```python
from build123d import *
from build123d.topology import SkipClean

# Parameters (mm, degrees)
SKETCH2_R           = 2.5
BOSS_EXTRUDE1_DEPTH = 7
FILLET1_R           = 90
BOSS_EXTRUDE3_DEPTH = 15
SKETCH4_R           = 8
CUT_EXTRUDE1_DEPTH  = 10
BOSS_EXTRUDE4_START = 10
BOSS_EXTRUDE4_DEPTH = 10
BOSS_EXTRUDE5_DEPTH = 27
SKETCH7_R           = 2.5
CUT_EXTRUDE2_DEPTH  = 37
INTERSECT3_DEPTH    = 27


with BuildPart() as part:
    # Sketch2 → Boss-Extrude1 (new body)
    with BuildSketch(Plane(origin=(0, 0, 0), x_dir=(1, 0, 0), z_dir=(0, 1, 0))):
        with BuildLine():
            Line((-4.24846021, -9.602113613), (13.572308451, -17.486922065))
            ThreePointArc((13.572308451, -17.486922065), (20.638500285, -15.805826469), (20.907079545, -8.547382103))
            Line((20.907079545, -8.547382103), (11.451696022, 4.891208687))
            ThreePointArc((11.451696022, 4.891208687), (9.270724445, 7.034926316), (6.472222222, 8.268031175))
            ThreePointArc((6.472222222, 8.268031175), (4.86754966, 9.30359932), (3.101845071, 10.031378627))
            Line((3.101845071, 10.031378627), (-8.821699821, 13.718308443))
            ThreePointArc((-8.821699821, 13.718308443), (-15.091857172, 11.987583677), (-16.147811194, 5.569231667))
            Line((-16.147811194, 5.569231667), (-12.308520784, -3.358124948))
            ThreePointArc((-12.308520784, -3.358124948), (-9.971976629, -6.504419403), (-6.472222222, -8.268031175))
            ThreePointArc((-6.472222222, -8.268031175), (-5.401685102, -9.003987898), (-4.24846021, -9.602113613))
        make_face()
        with Locations(Location((16, -12, 0), (0, 0, 270))):
            Circle(SKETCH2_R, mode=Mode.SUBTRACT)
        with Locations(Location((-10.604337088, 7.953252816, 0), (0, 0, 270))):
            Circle(SKETCH2_R, mode=Mode.SUBTRACT)
        with BuildLine():
            ThreePointArc((-4.694444444, -4.495797077), (0, -6.5), (4.694444444, -4.495797077))
            ThreePointArc((4.694444444, -4.495797077), (9, 0), (4.694444444, 4.495797077))
            ThreePointArc((4.694444444, 4.495797077), (0, 6.5), (-4.694444444, 4.495797077))
            ThreePointArc((-4.694444444, 4.495797077), (-9, 0), (-4.694444444, -4.495797077))
        make_face(mode=Mode.SUBTRACT)
    extrude(amount=BOSS_EXTRUDE1_DEPTH)

    # Fillet1
    fillet1_edges = [part.edges().sort_by_distance(p)[0] for p in [
        (6.472222222, 3.5, -8.268031175),
        (-6.472222222, 3.5, 8.268031175),
    ]]
    fillet(fillet1_edges, radius=FILLET1_R)

    # Sketch3 → Boss-Extrude3 (add)
    with BuildSketch(Plane(origin=(0, 7, 0), x_dir=(1, 0, 0), z_dir=(0, 1, 0))):
        with BuildLine():
            Line((-13.446880098, 1.012795393), (-12.308520784, -3.358124948))
            ThreePointArc((-12.308520784, -3.358124948), (-10.611843956, -5.907229762), (-8.121968415, -7.689690813))
            ThreePointArc((-8.121968415, -7.689690813), (-6.480430757, -8.483296944), (-4.855306799, -9.309994408))
            ThreePointArc((-4.855306799, -9.309994408), (-4.554226262, -9.460920841), (-4.24846021, -9.602113613))
            Line((-4.24846021, -9.602113613), (-1.454246479, -10.838414946))
            ThreePointArc((-1.454246479, -10.838414946), (10.979115699, -7.880432641), (11.451696022, 4.891208687))
            ThreePointArc((11.451696022, 4.891208687), (9.968863726, 6.507036925), (8.121968415, 7.689690813))
            ThreePointArc((8.121968415, 7.689690813), (6.480430757, 8.483296944), (4.855306799, 9.309994408))
            ThreePointArc((4.855306799, 9.309994408), (3.994892398, 9.710346787), (3.101845071, 10.031378627))
            Line((3.101845071, 10.031378627), (-3.895223267, 11.305534387))
            ThreePointArc((-3.895223267, 11.305534387), (-5.691953988, 10.727471116), (-6.207623157, 8.911848981))
            ThreePointArc((-6.207623157, 8.911848981), (-7.30582589, 4.892236012), (-11.232333003, 3.497288147))
            ThreePointArc((-11.232333003, 3.497288147), (-13.004436636, 2.847636589), (-13.446880098, 1.012795393))
        make_face()
        with BuildLine():
            ThreePointArc((4.694444444, -4.495797077), (9, 0), (4.694444444, 4.495797077))
            ThreePointArc((4.694444444, 4.495797077), (0, 6.5), (-4.694444444, 4.495797077))
            ThreePointArc((-4.694444444, 4.495797077), (-9, 0), (-4.694444444, -4.495797077))
            ThreePointArc((-4.694444444, -4.495797077), (0, -6.5), (4.694444444, -4.495797077))
        make_face(mode=Mode.SUBTRACT)
    extrude(amount=BOSS_EXTRUDE3_DEPTH)

    # Sketch4 → Cut-Extrude1 (cut)
    with BuildSketch(Plane(origin=(0, 22, 0), x_dir=(1, 0, 0), z_dir=(0, 1, 0))):
        Circle(SKETCH4_R)
    extrude(amount=-CUT_EXTRUDE1_DEPTH, mode=Mode.SUBTRACT)

    # Sketch5 → Boss-Extrude4 (add)
    with SkipClean():  # the faces are left unmerged after this step: merging them gives an invalid solid
        with BuildSketch(Plane(origin=(0, 12, 0), x_dir=(1, 0, 0), z_dir=(0, 1, 0)).offset(BOSS_EXTRUDE4_START)):
            with BuildLine():
                ThreePointArc((-7.111111111, 3.664982778), (-8, 0), (-7.111111111, -3.664982778))
                ThreePointArc((-7.111111111, -3.664982778), (-9, 0), (-7.111111111, 3.664982778))
            make_face()
            with BuildLine():
                ThreePointArc((7.111111111, -3.664982778), (9, 0), (7.111111111, 3.664982778))
                ThreePointArc((7.111111111, 3.664982778), (8, 0), (7.111111111, -3.664982778))
            make_face()
        extrude(amount=-BOSS_EXTRUDE4_DEPTH)


with BuildPart() as body_2:
    # Sketch6 → Boss-Extrude5 (new body)
    with BuildSketch(Plane(origin=(0, 0, 0), x_dir=(-1, 0, 0), z_dir=(0, -1, 0))):
        Polygon((8.401052482, 26.937158796), (-31.729302738, -9.377746691), (-13.016359271, -30.388770935), (27.113995949, 5.926134553), align=None)
    extrude(amount=-BOSS_EXTRUDE5_DEPTH)

    # Sketch7 → Cut-Extrude2 (cut)
    with BuildSketch(Plane(origin=(-9.25873614, 0, 10.23151142), x_dir=(0.7414761288495602, 0, 0.670979247329059), z_dir=(-0.670979247329059, 0, 0.7414761288495602))):
        with Locations((-16.542969249, 20.228212297)):
            Circle(SKETCH7_R)
        with Locations((19.254983261, 20.228212297)):
            Circle(SKETCH7_R)
    extrude(amount=-CUT_EXTRUDE2_DEPTH, mode=Mode.SUBTRACT)

    # Intersect1: read off the stored shape, not the designer's step
    # Intersect1: cut part
    add(part.part, mode=Mode.SUBTRACT)

    # Intersect3: read off the stored shape, not the designer's step
    # Intersect3 outline → Intersect3 (cut)
    with BuildSketch(Plane(origin=(0, 0, 0), x_dir=(1, 0, 0), z_dir=(0, 1, 0))):
        Polygon((13.016359271, -30.388770935), (22.372831004, -19.883258813), (-17.757524216, 16.431646675), (-27.113995949, 5.926134553), align=None)
    extrude(amount=INTERSECT3_DEPTH, mode=Mode.SUBTRACT)


solid = body_2.part
```
Can you work these out from the model? Positions are in its coordinate system, mm. A direction names the side the tool comes from. Round coordinates to 2 decimals unless told otherwise and drop trailing zeros. Loops run counter-clockwise (first coordinate to the right, second up) from the corner with the lowest first, then second, coordinate; pieces in that order, holes last. Notation, with made-up numbers: (56, 32) -> (108, 32) arc R15 ccw to (108, 38) -> close; hole circle Ø6 at (19, -40). An arc over 180 degrees is marked (long way). One line per item, written item: value. Start each with the question number.
1. If we mould it in two halves opening along Y, with no side actions, what happens to faces 3 (the flat face through (7, 0, -9)), 4 (the cylindrical face through (17.735, 3.451, 10.2)), 5 (the cylindrical face through (-7.834, 17.788, -16.805)), 6 (the cylindrical face through (20.82, 19.27, 9.13))? For each: pulls with the +Y half, pulls with the -Y half, needs draft (parallel to the pull), parting line crosses it, or undercut.
2. If we section it at B-B, the plane z = -3: Write out the boundary of the cut face in (x, y), then the cut area to 3 significant figures.
3. If we section it at A-A, the plane y = 16: Write out the boundary of the cut face in (x, z).
4. If we section it at C-C, the plane y = 5.75: Give the number of separate pieces and of enclosed holes in the cut face, then the cut area to 3 significant figures.
5. For faces 1 (the flat face through (27.117, 13.311, 14.557)), 2 (the cylindrical face through (6.503, 14.395, -8.472)), which set-ups out of +Z, -Z, +X, -X, +Y, -Y let a thin tool reach every point of the face, with its end or its side?
6. For pin 1 (5 mm diameter, centred on y = 3, z = -5.5, fed in from -X); pin 2 (8 mm diameter, centred on x = -3.5, y = 21.5, fed in from -Z); pin 3 (10 mm diameter, centred on x = -3, y = 22.5, fed in from -Z); pin 4 (6 mm diameter, centred on x = 17, z = 1, fed in from -Y), each with a flat end and sliding along its axis, tell me the tip position at first contact or that it passes through.
7. If I drill on probe 1 along Z at (x, y) = (11, 12); probe 2 along X at (y, z) = (12.75, 2.5); probe 3 along X at (y, z) = (4.5, 14), over which ranges is the centre line in solid material (lowest first)?
Calculated:
1. face 3: pulls with the -Y half
1. face 4: needs draft
1. face 5: undercut
1. face 6: undercut
2. outline: (-2.91, 0) -> (7.85, 0) -> (7.85, 12) -> (7.42, 12) -> (7.42, 22) -> (12.51, 22) -> (12.51, 7) -> (12.78, 7) -> (12.78, 0) -> (18.05, 0) -> (18.05, 27) -> (-2.91, 27) -> close
2. area: 457 mm²
3. outline: (-17.76, -16.43) -> (-8.4, -26.94) -> (31.73, 9.38) -> (22.37, 19.88) -> (10.13, 8.8) arc R10.56 cw to (11.45, -4.89) arc R8.5 cw to (8.12, -7.69) arc R90 ccw to (4.86, -9.31) arc R10.5 cw to (3.1, -10.03) -> (-3.9, -11.31) arc R2 cw to (-6.21, -8.91) arc R4.5 ccw to (-6.46, -6.21) -> close; (-5.75, -5.56) arc R8 ccw to (6.11, 5.17) -> close
4. separate pieces: 4
4. enclosed holes: 0
4. area: 502 mm²
5. face 1: +Z, +X, +Y, -Y
5. face 2: -Y
6. pin 1: stops at x = -8.44
6. pin 2: stops at z = -26.12
6. pin 3: stops at z = -26.57
6. pin 4: stops at y = 0
7. probe 1: z = -9.38 to -5.48, 7.85 to 9.59
7. probe 2: x = 3.16 to 7.6, 13.29 to 24.13
7. probe 3: x = 15.87 to 17.5, 21.66 to 27.61
